Design review of the part built by this model. Coordinates are the model's own, in mm. Face numbers are marked on the shaded views. A direction names the side the tool comes from. Give positions to 0.01 mm unless a question says otherwise; leave off trailing zeros. Write each loop counter-clockwise with the first axis right and the second up, starting at its lowest first coordinate (ties: lowest second). Pieces come first, ordered by that corner, then holes. Notation, with made-up numbers: M 55.25,-6.5 L 93.25,-6.5 A31 ccw 93.25,29.5 Z; hole C -25,-28 d8. An arc over 180 degrees is marked long. Use a Markdown table: item, result. Add a question column.
```python
from build123d import *

# Parameters (mm, degrees)
SKETCH_1_W           = 40
SKETCH_1_H           = 85
EXTRUDE_1_DEPTH      = 20
SKETCH_2_W           = 30
SKETCH_2_H           = 60
CUT_EXTRUDE_1_DEPTH  = 15
SKETCH_3_W           = 31.5
SKETCH_3_H           = 16
CUT_EXTRUDE_3_DEPTH  = 7
SKETCH_4_R           = 1.5
CUT_EXTRUDE_4_DEPTH  = 16
FILLET_1_R           = 2
FILLET_2_R           = 2
SKETCH_6_W           = 15.3
SKETCH_6_H           = 12
CUT_EXTRUDE_5_DEPTH  = 4
SKETCH_7_W           = 3
SKETCH_7_H           = 52
EXTRUDE_2_DEPTH      = 10
SKETCH_8_W           = 17
SKETCH_8_H           = 1.5
CUT_EXTRUDE_6_DEPTH  = 2
CHAMFER_1_SIZE       = 0.7
SKETCH_9_R           = 3
CUT_EXTRUDE_7_DEPTH  = 15
SKETCH_10_W          = 3
SKETCH_10_H          = 3
CUT_EXTRUDE_8_DEPTH  = 2.5
EXTRUDE_START        = -15
SKETCH_14_R          = 6.25
EXTRUDE_4_DEPTH      = 10
CUT_EXTRUDE_START    = -5
SKETCH_16_R          = 5
CUT_EXTRUDE_10_DEPTH = 5
SKETCH_17_R          = 1.8
CUT_EXTRUDE_11_DEPTH = 96.131487952
CUT_EXTRUDE_12_DEPTH = 12


with BuildPart() as part:
    # Эскиз1 → Бобышка-Вытянуть1 (new body)
    with BuildSketch(Plane.XY):
        with Locations((-20, -42.5)):
            Rectangle(SKETCH_1_W, SKETCH_1_H)
    extrude(amount=EXTRUDE_1_DEPTH)

    # Эскиз2 → Вырез-Вытянуть1 (cut)
    with BuildSketch(Plane(origin=(0, 0, 0), x_dir=(-1, 0, 0), z_dir=(0, 0, -1))):
        with Locations((20, -36)):
            Rectangle(SKETCH_2_W, SKETCH_2_H)
    extrude(amount=-CUT_EXTRUDE_1_DEPTH, mode=Mode.SUBTRACT)

    # Эскиз3 → Вырез-Вытянуть3 (cut)
    with BuildSketch(Plane.XZ.offset(85)):
        with Locations((-20, 8)):
            Rectangle(SKETCH_3_W, SKETCH_3_H)
    extrude(amount=-CUT_EXTRUDE_3_DEPTH, mode=Mode.SUBTRACT)

    # Эскиз4 → Вырез-Вытянуть4 (cut)
    with BuildSketch(Plane.XZ.offset(78)):
        with Locations(Location((-7.5, 9.636214897, 0), (0, 0, 270))):
            Circle(SKETCH_4_R)
        with Locations(Location((-32.5, 9.636214897, 0), (0, 0, 270))):
            Circle(SKETCH_4_R)
        with BuildLine():
            Line((-13.531390771, 15.3), (-26.468609229, 15.3))
            ThreePointArc((-26.468609229, 15.3), (-28.268414536, 14.644924441), (-29.226070938, 12.986214897))
            Line((-29.226070938, 12.986214897), (-30.407461708, 6.286214897))
            ThreePointArc((-30.407461708, 6.286214897), (-29.794924441, 4.000194693), (-27.65, 3))
            Line((-27.65, 3), (-12.35, 3))
            ThreePointArc((-12.35, 3), (-10.205075559, 4.000194693), (-9.592538292, 6.286214897))
            Line((-9.592538292, 6.286214897), (-10.773929062, 12.986214897))
            ThreePointArc((-10.773929062, 12.986214897), (-11.731585464, 14.644924441), (-13.531390771, 15.3))
        make_face()
    extrude(amount=-CUT_EXTRUDE_4_DEPTH, mode=Mode.SUBTRACT)

    # Скругление1
    fillet_1_edges = [part.edges().sort_by_distance(p)[0] for p in [
        (-4.25, -81.5, 16),
        (-35.75, -81.5, 16),
    ]]
    fillet(fillet_1_edges, radius=FILLET_1_R)

    # Скругление2
    fillet_2_edges = [part.edges().sort_by_distance(p)[0] for p in [
        (0, -85, 10),
        (-40, -85, 10),
        (-40, 0, 10),
        (0, 0, 10),
    ]]
    fillet(fillet_2_edges, radius=FILLET_2_R)

    # Эскиз6 → Вырез-Вытянуть5 (cut)
    with BuildSketch(Plane(origin=(0, 0, 0), x_dir=(-1, 0, 0), z_dir=(0, 0, -1))):
        with Locations((20, -72)):
            Rectangle(SKETCH_6_W, SKETCH_6_H)
    extrude(amount=-CUT_EXTRUDE_5_DEPTH, mode=Mode.SUBTRACT)

    # Эскиз7 → Бобышка-Вытянуть2 (add)
    with BuildSketch(Plane(origin=(0, 0, 15), x_dir=(-1, 0, 0), z_dir=(0, 0, -1))):
        with Locations((10.1, -32)):
            Rectangle(SKETCH_7_W, SKETCH_7_H)
        with Locations((27.1, -32)):
            Rectangle(SKETCH_7_W, SKETCH_7_H)
    extrude(amount=EXTRUDE_2_DEPTH)

    # Эскиз8 → Вырез-Вытянуть6 (cut)
    with BuildSketch(Plane.XZ.offset(6)):
        with Locations((-18.6, 4.25)):
            Rectangle(SKETCH_8_W, SKETCH_8_H)
    extrude(amount=-CUT_EXTRUDE_6_DEPTH, mode=Mode.SUBTRACT)

    # Фаска1
    chamfer_1_edges = [part.edges().sort_by_distance(p)[0] for p in [
        (-18.6, -4, 3.5),
    ]]
    chamfer(chamfer_1_edges, length=CHAMFER_1_SIZE)

    # Эскиз9 → Вырез-Вытянуть7 (cut)
    with BuildSketch(Plane.XZ.offset(6)):
        with Locations(Location((-20, 10.022807371, 0), (0, 0, 270))):
            Circle(SKETCH_9_R)
    extrude(amount=-CUT_EXTRUDE_7_DEPTH, mode=Mode.SUBTRACT)

    # Эскиз10 → Вырез-Вытянуть8 (cut)
    with BuildSketch(Plane(origin=(0, -66, 0), x_dir=(1, 0, 0), z_dir=(0, 1, 0))):
        with Locations((-33.5, -3.5)):
            Rectangle(SKETCH_10_W, SKETCH_10_H)
        with Locations((-6.5, -3.5)):
            Rectangle(SKETCH_10_W, SKETCH_10_H)
    extrude(amount=-CUT_EXTRUDE_8_DEPTH, mode=Mode.SUBTRACT)

    # Эскиз14 → Бобышка-Вытянуть4 (add)
    with BuildSketch(Plane(origin=(0, 0, 0), x_dir=(-1, 0, 0), z_dir=(0, 0, -1)).offset(EXTRUDE_START)):
        with Locations((6.25, -6.25)):
            Circle(SKETCH_14_R)
        with Locations((33.75, -6.25)):
            Circle(SKETCH_14_R)
    extrude(amount=EXTRUDE_4_DEPTH)

    # Эскиз16 → Вырез-Вытянуть10 (cut)
    with BuildSketch(Plane(origin=(0, 0, 0), x_dir=(-1, 0, 0), z_dir=(0, 0, -1)).offset(CUT_EXTRUDE_START)):
        with Locations((6.25, -6.25)):
            Circle(SKETCH_16_R)
        with Locations((33.75, -6.25)):
            Circle(SKETCH_16_R)
    extrude(amount=CUT_EXTRUDE_10_DEPTH, mode=Mode.SUBTRACT)

    # Эскиз17 → Вырез-Вытянуть11 (cut, through all)
    with BuildSketch(Plane(origin=(0, 0, 5), x_dir=(-1, 0, 0), z_dir=(0, 0, -1))):
        with Locations((6.25, -6.25)):
            Circle(SKETCH_17_R)
        with Locations((33.75, -6.25)):
            Circle(SKETCH_17_R)
    extrude(amount=-CUT_EXTRUDE_11_DEPTH, mode=Mode.SUBTRACT)

    # Эскиз18 → Вырез-Вытянуть12 (cut)
    with BuildSketch(Plane.XY.offset(20)):
        Polygon((-6.25, -9.714101615), (-3.25, -7.982050808), (-3.25, -4.517949192), (-6.25, -2.785898385), (-9.25, -4.517949192), (-9.25, -7.982050808), align=None)
        Polygon((-30.75, -4.517949192), (-33.75, -2.785898385), (-36.75, -4.517949192), (-36.75, -7.982050808), (-33.75, -9.714101615), (-30.75, -7.982050808), align=None)
    extrude(amount=-CUT_EXTRUDE_12_DEPTH, mode=Mode.SUBTRACT)


solid = part.part
```
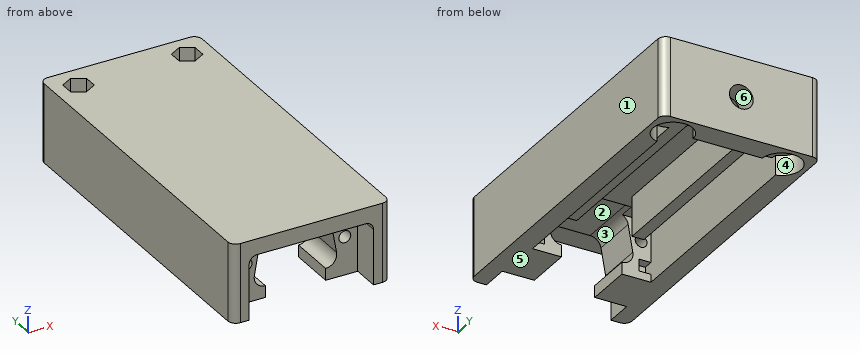
(1) Add section C-C on y = -52. Give the boundary of the cut face in (x, z).
(2) Add section B-B on x = -20. Give the boundary of the cut face in (y, z), then the cut area to 3 significant figures.
(3) The part is to be moulded in two halves that separate along Z. For the marked faces 4, 5 and 6, say which applies: released by +Z, released by -Z, zero draft, split by the parting line, or undercut.
(4) Wall thickness on L1, parallel to X at y = -52, z = 7; L2, parallel to Y at x = -6.25, z = 5.95; L3, parallel to X at y = -59.5, z = 14: over which ranges is each line inside the solid? List them lowest first.
(5) Add section D-D on z = 10.25. Give the number of separate pieces and of enclosed holes in the cut face, then the cut area to 3 significant figures.
(6) Add section A-A on z = 17. Give the boundary of the cut face in (x, y), then the cut area to 3 significant figures.
(7) For pin 1 (1 mm diameter, centred on x = -23, y = -63.5, fed in from -Z); pin 2 (4 mm diameter, centred on x = -6.25, y = -6.25, fed in from +Z); pin 3 (5 mm diameter, centred on x = -32.5, z = 9.64, fed in from -Y), all flat-tipped, find the tip position at first contact; note any pin that passes through.
(8) Machinability: for the marked faces 1, 2 and 3, which of the approach directions +Z, -Z, +X, -X, +Y, -Y give a long, thin tool a straight path to every point of the face, cutting with its end or side? Answer none if there is none.
From the geometry:
| question | item | result |
|---|---|---|
| 1 | outline | M -40,0 L -35,0 L -35,15 L -28.6,15 L -28.6,5 L -25.6,5 L -25.6,15 L -11.6,15 L -11.6,5 L -8.6,5 L -8.6,15 L -5,15 L -5,0 L 0,0 L 0,20 L -40,20 Z |
| 2 | outline | M -85,16 L -78,16 L -78,15.3 L -62,15.3 L -62,15 L -6,15 L -6,13.02 L 0,13.02 L 0,20 L -85,20 Z; M -6,0 L 0,0 L 0,7.02 L -6,7.02 L -6,5 L -4,5 L -4,4.2 L -4.7,3.5 L -6,3.5 Z |
| 2 | area | 464 mm^2 |
| 3 | face 4 | zero draft |
| 3 | face 5 | released by -Z |
| 3 | face 6 | undercut |
| 4 | L1 | x = -40 to -35, -28.6 to -25.6, -11.6 to -8.6, -5 to 0 |
| 4 | L2 | y = -78 to -66, -12.5 to -8.05, -4.45 to 0 |
| 4 | L3 | x = -40 to -35, -5 to 0 |
| 5 | separate pieces | 4 |
| 5 | enclosed holes | 2 |
| 5 | area | 1,350 mm^2 |
| 6 | outline | M -40,-83 A2 ccw -38,-85 L -2,-85 A2 ccw 0,-83 L 0,-2 A2 ccw -2,0 L -38,0 A2 ccw -40,-2 Z; hole M -36.75,-7.98 L -33.75,-9.71 L -30.75,-7.98 L -30.75,-4.52 L -33.75,-2.79 L -36.75,-4.52 Z; hole M -9.25,-7.98 L -6.25,-9.71 L -3.25,-7.98 L -3.25,-4.52 L -6.25,-2.79 L -9.25,-4.52 Z |
| 6 | area | 3,330 mm^2 |
| 7 | pin 1 | stops at z = 15.3 |
| 7 | pin 2 | stops at z = 8 |
| 7 | pin 3 | stops at y = -78 |
| 8 | face 1 | +Z, -Z, +X, +Y, -Y |
| 8 | face 2 | -Z, -Y |
| 8 | face 3 | -Y |
